```python
from build123d import *

# Parameters (mm, degrees)
ESBO_O1_R                     = 50
RESSALTO_EXTRUS_O1_DEPTH      = 26.75
RESSALTO_EXTRUS_O3_REACH      = 141.085
RESSALTO_EXTRUS_O3_END_RADIUS = 50
ESBO_O2_R                     = 32.5
ESBO_O3_R                     = 26.25
RESSALTO_EXTRUS_O4_DEPTH      = 5
ESBO_O4_R                     = 6
CORTE_EXTRUS_O1_DEPTH         = 113.8475189


with BuildPart() as part:
    # Esboço1 → Ressalto-extrusão1 (new, symmetric)
    with BuildSketch(Plane.XY):
        Circle(ESBO_O1_R)
    extrude(amount=RESSALTO_EXTRUS_O1_DEPTH, both=True)

    # Ressalto-extrusão3: up to this cylinder (the profile starts outside it)
    ressalto_extrus_o3_end = Plane(origin=(0, 0, 0), z_dir=(0, 0, -1)) * Cylinder(RESSALTO_EXTRUS_O3_END_RADIUS, 383.17, mode=Mode.PRIVATE)
    # Esboço2 → Ressalto-extrusão3 (add, up to the surface)
    with BuildSketch(Plane(origin=(77, 0, 0), x_dir=(0, 0, -1), z_dir=(1, 0, 0)), mode=Mode.PRIVATE) as ressalto_extrus_o3_sk1:
        Circle(ESBO_O2_R)
    ressalto_extrus_o3_tool1 = extrude(ressalto_extrus_o3_sk1.sketch, amount=-RESSALTO_EXTRUS_O3_REACH, mode=Mode.PRIVATE) - ressalto_extrus_o3_end
    add(ressalto_extrus_o3_tool1.solids().sort_by_distance((77, 0, 0))[0])

    # Esboço3 → Ressalto-extrusão4 (add)
    with BuildSketch(Plane(origin=(77, 0, 0), x_dir=(0, 0, -1), z_dir=(1, 0, 0))):
        Circle(ESBO_O3_R)
    extrude(amount=RESSALTO_EXTRUS_O4_DEPTH)

    # Esboço4 → Corte-extrusão1 (cut, through all)
    with BuildSketch(Plane.XY.offset(26.75)):
        Circle(ESBO_O4_R)
    extrude(amount=-CORTE_EXTRUS_O1_DEPTH, mode=Mode.SUBTRACT)


solid = part.part
```
Work out the finished part from the listing and answer in its coordinate system (mm). A direction names the side the tool comes from. Coordinates: 2 decimals unless noted, no trailing zeros. Loops run counter-clockwise (first coordinate to the right, second up) from the corner with the lowest first, then second, coordinate; pieces in that order, holes last. Notation, with made-up numbers: (12.5, 13.5) -> (67.5, 13.5) arc R15 ccw to (67.5, 35.5) -> close; hole circle Ø8 at (-14.75, -35). An arc over 180 degrees is marked (long way). Answer as CSV lines item,"result".
Q1. The part is cut by section C-C on z = 0. Write down the section's boundary in (x, y).
Findings:
outline,"(38, -32.5) -> (77, -32.5) -> (77, -26.25) -> (82, -26.25) -> (82, 26.25) -> (77, 26.25) -> (77, 32.5) -> (38, 32.5) arc R50 ccw (long way) to start; hole circle Ø12 at (0, 0)"
Q2. The part is cut by section A-A on y = 0. Write down the section's boundary in (x, z), and give its area (3 significant figures).
Findings:
outline,"(-50, -26.75) -> (-6, -26.75) -> (-6, 26.75) -> (-50, 26.75) -> close; (6, -26.75) -> (50, -26.75) -> (50, -32.5) -> (77, -32.5) -> (77, -26.25) -> (82, -26.25) -> (82, 26.25) -> (77, 26.25) -> (77, 32.5) -> (50, 32.5) -> (50, 26.75) -> (6, 26.75) -> close"
area,"6,730 mm²"
Q3. Find the intervals of material crossed by probe 1 along Y at (x, z) = (0, 11); probe 2 along Z at (x, y) = (8, 1), in increasing order.
Findings:
probe 1,"y = -50 to -6, 6 to 50"
probe 2,"z = -26.75 to 26.75"
Q4. The part is cut by section B-B on x = 0. Write down the section's boundary in (y, z), and give its area (3 significant figures).
Findings:
outline,"(-50, -26.75) -> (-6, -26.75) -> (-6, 26.75) -> (-50, 26.75) -> close; (6, -26.75) -> (50, -26.75) -> (50, 26.75) -> (6, 26.75) -> close"
area,"4,710 mm²"
Q5. The part is cut by section D-D on y = 23. Write down the section's boundary in (x, z), and give its area (3 significant figures).
Findings:
outline,"(-44.4, -26.75) -> (44.4, -26.75) -> (44.4, -22.96) -> (77, -22.96) -> (77, -12.65) -> (82, -12.65) -> (82, 12.65) -> (77, 12.65) -> (77, 22.96) -> (44.4, 22.96) -> (44.4, 26.75) -> (-44.4, 26.75) -> close"
area,"6,370 mm²"
Q6. For a pull along X with two mould halves and no side action, classify faces 4 (the face through (50, 0, -29)), 5 (the face through (-6, 0, 0)), 6 (the face through (-1, -10, -26.75)) as +X half, -X half, draft (parallel to the pull), parting line (faces both ways), or undercut.
Findings:
face 4,"-X half"
face 5,"undercut"
face 6,"draft"
Q7. A tool of negligible diameter and unlimited length cuts with its end or side. For faces 1 (the face through (50, 0, 29)), 2 (the face through (79, 8, -25)), 3 (the face through (82, 0, 0)), from which of +Z, -Z, +X, -X, +Y, -Y can it reach the whole face along a straight path? Write none if from no direction.
Findings:
face 1,"+Z, -X"
face 2,"+X"
face 3,"+Z, -Z, +X, +Y, -Y"
Q8. Each of these flat-tipped pins is pushed along its axis until it touches: pin 1 (1 mm diameter, centred on x = 22, z = -8, fed in from +Y); pin 2 (5 mm diameter, centred on y = -38.5, z = 25.5, fed in from +X); pin 3 (5 mm diameter, centred on y = 27, z = -12.5, fed in from +X). Where does it stop, or does it pass through?
Findings:
pin 1,"stops at y = 45.14"
pin 2,"stops at x = 34.7"
pin 3,"stops at x = 77"
